Check sheet for the drawn part. Datum: minimum x, y, z corner. Units: mm. Give positions to 0.01 mm unless a question says otherwise; leave off trailing zeros. Write each loop counter-clockwise with the first axis right and the second up, starting at its lowest first coordinate (ties: lowest second). Pieces come first, ordered by that corner, then holes. Notation, with made-up numbers: M -4.75,0 L 32.25,0 A21 cw 32.25,32 Z; hole C 57,86.25 d7. An arc over 180 degrees is marked long. Write item = value, one per line.
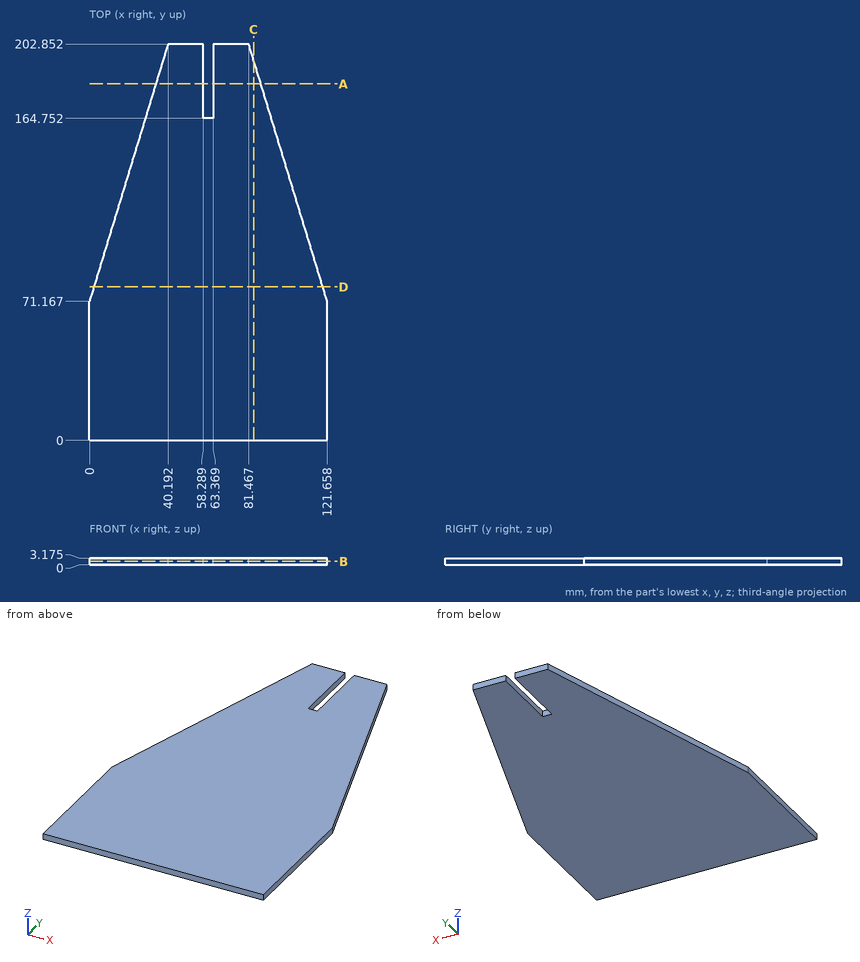
1) Material ranges on probe 1 along X at (y, z) = (190.5, 2.8); probe 2 along X at (y, z) = (170, 2.9) (1 decimal); probe 3 along X at (y, z) = (156, 2.6), recorded low to high. Write a range as from..to.
From the geometry:
probe_1 = 36.42..58.29, 63.37..85.24
probe_2 = 30.2..58.3, 63.4..91.5
probe_3 = 25.89..95.77
2) Depth check by flat-ended pin: P1, Ø1, axis at x = 65, y = 107.5, coming from the -Z side; P2, Ø1, axis at y = 191.5, z = 2, coming from the -X side (1 decimal); P3, Ø1.6, axis at y = 190.5, z = 2, coming from the +X side. Enter the tip coordinate at first touch or a pass-through.
From the geometry:
P1 = 0
P2 = 36.6
P3 = 85.48
3) Cross-section at B-B on z = 1.65. Record the boundary of the cut face in (x, y), plus the area to 3 significant figures.
From the geometry:
outline = M 0,0 L 121.66,0 L 121.66,71.17 L 81.47,202.85 L 63.37,202.85 L 63.37,164.75 L 58.29,164.75 L 58.29,202.85 L 40.19,202.85 L 0,71.17 Z
area = 19,200 mm^2
4) Cross-section at D-D on y = 78.5. Record the boundary of the cut face in (x, z) (1 decimal), plus the area to 3 significant figures.
From the geometry:
outline = M 2.2,0 L 119.4,0 L 119.4,3.2 L 2.2,3.2 Z
area = 372 mm^2
5) Cross-section at A-A on y = 182.5. Record the boundary of the cut face in (x, z) (1 decimal).
From the geometry:
outline = M 34,0 L 58.3,0 L 58.3,3.2 L 34,3.2 Z; M 63.4,0 L 87.7,0 L 87.7,3.2 L 63.4,3.2 Z
6) Cross-section at C-C on x = 84. Record the boundary of the cut face in (y, z) (1 decimal).
From the geometry:
outline = M 0,0 L 194.6,0 L 194.6,3.2 L 0,3.2 Z
